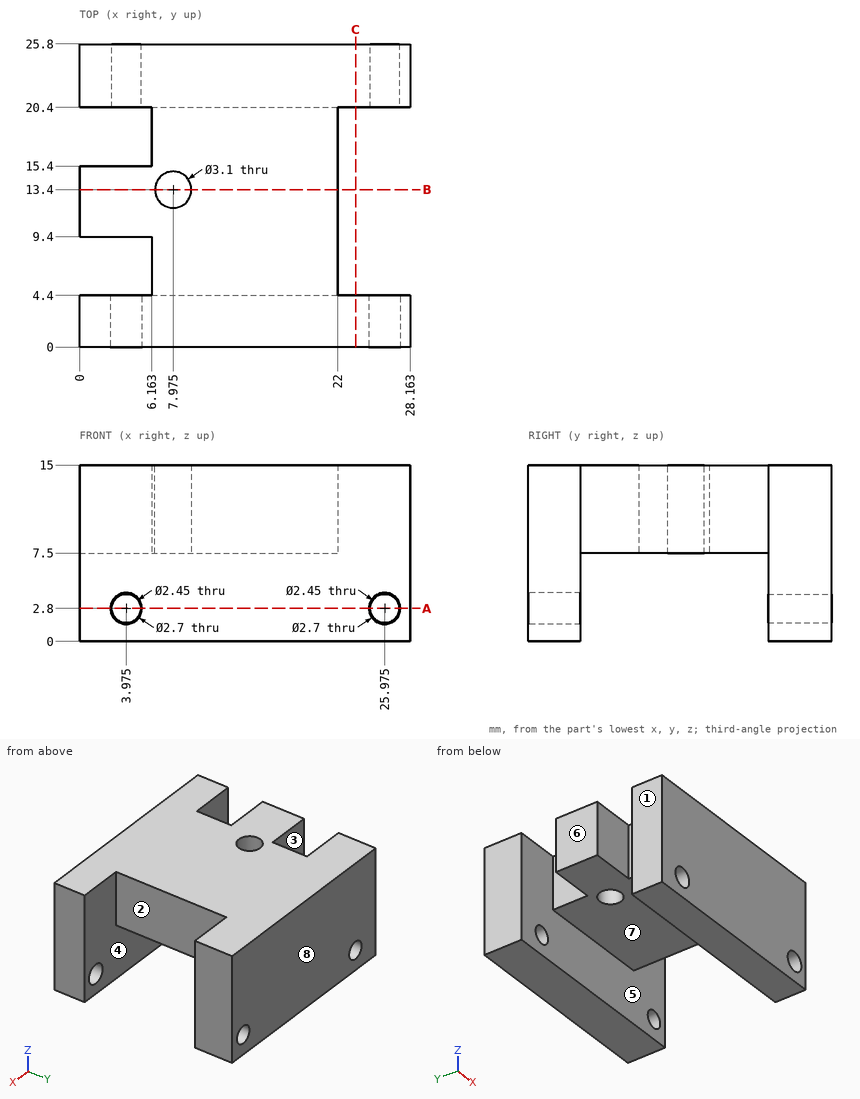
Print and shaded views of the part. All mm, measured from the part's lowest x, y and z. A direction names the side the tool comes from. Coordinates: 2 decimals unless noted, no trailing zeros. Order: outer loops, then holes, each group sorted by start corner. A loop starts at its lowest first (then second) coordinate and runs counter-clockwise, first axis right, second up. Notation, with made-up numbers: (2, -35.5) - (27, -35.5) arc R7 ccw to (27, -29.5) - close; hole circle Ø1 at (74.25, 39.5). An arc over 180 degrees is marked (long way). Return JSON: item names as keys, results as strings. Group by question number.
Item 1: Cut at B-B (y = 13.4). List the corners of the cut face in (x, z) (1 decimal), plus the area to 3 significant figures.
Item 2: Cut at A-A (z = 2.8). State how many separate pieces and enclosed holes the cut face has, plus the area to 3 significant figures.
Item 3: Which spindle directions (+Z, -Z, +X, -X, +Y, -Y) get a long thin tool onto all of the face, cutting with end or side? Do the marked faces 1, 2, 3 and 4. Say none if no direction does.
Item 4: Pin check, flat tips, straight feed: pin 1 (2 mm diameter, centred on y = 5.5, z = 2, fed in from +X); pin 2 (8 mm diameter, centred on y = 14.5, z = 11.5, fed in from +X); pin 3 (1.5 mm diameter, centred on y = 7, z = 10, fed in from -X); pin 4 (8 mm diameter, centred on x = 8.5, y = 14.5, fed in from -Z). Stop position of each tip, or through.
Item 5: Pull direction Y, two halves, no side cores. Call the marked faces 5, 6, 7 and 8: pulls with the +Y half, pulls with the -Y half, needs draft (parallel to the pull), parting line crosses it, or undercut.
Item 6: Drill centre lines: probe 1 along Y at (x, z) = (5.25, 11.75); probe 2 along X at (y, z) = (22.05, 2.8); probe 3 along Y at (x, z) = (10.5, 3.75). Where is each one in solid material? Low to high. Write a range as from..to.
Item 7: Cut at C-C (x = 23.5). List the corners of the cut face in (y, z).
Check values:
{
 "1": {"outline": "(0, 7.5) - (6.4, 7.5) - (6.4, 15) - (0, 15) - close; (9.5, 7.5) - (22, 7.5) - (22, 15) - (9.5, 15) - close", "area": "142 mm2"},
 "2": {"separate pieces": "6", "enclosed holes": "0", "area": "226 mm2"},
 "3": {"face 1": "+Z, -Z, -X, +Y, -Y", "face 2": "+Z, -Z, +X", "face 3": "+Z, -Z, -X", "face 4": "-Z"},
 "4": {"pin 1": "passes through", "pin 2": "stops at x = 22", "pin 3": "stops at x = 6.16", "pin 4": "stops at z = 7.5"},
 "5": {"face 5": "undercut", "face 6": "needs draft", "face 7": "undercut", "face 8": "pulls with the +Y half"},
 "6": {"probe 1": "y = 0..4.4, 9.4..15.4, 20.4..25.8", "probe 2": "x = 0..2.75, 5.2..24.75, 27.2..28.16", "probe 3": "y = 0..4.4, 20.4..25.8"},
 "7": {"outline": "(0, 0) - (4.4, 0) - (4.4, 15) - (0, 15) - close; (20.4, 0) - (25.8, 0) - (25.8, 15) - (20.4, 15) - close"}
}
